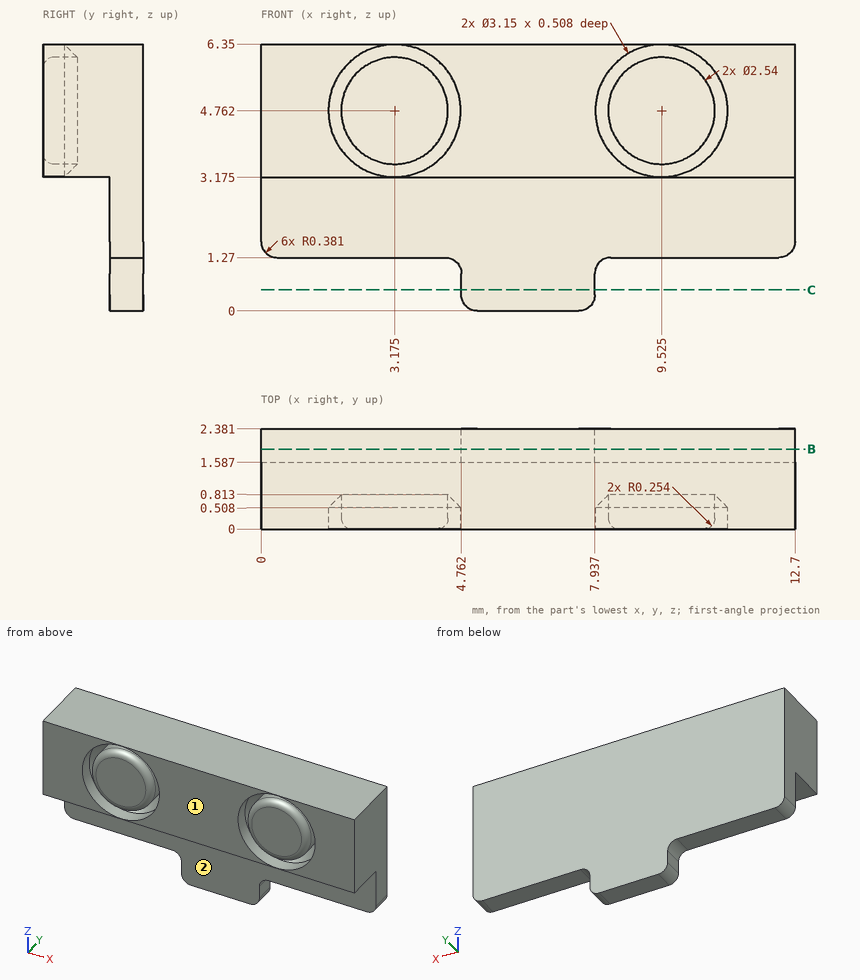
Could you check a few things on this drawing? It's one solid part, dimensions in mm from its lowest x, y, z. A direction names the side the tool comes from. Round coordinates to 2 decimals unless told otherwise and drop trailing zeros. Write each loop counter-clockwise with the first axis right and the second up, starting at its lowest first coordinate (ties: lowest second). Pieces come first, ordered by that corner, then holes. Notation, with made-up numbers: (-1.5, -22) -> (39.5, -22) arc R29 cw to (39.5, 12) -> close; hole circle Ø9 at (51, 56.5). An arc over 180 degrees is marked (long way). One line per question, with ' | ' between items. Start each with the question number.
1) On a 3-axis mill with a long thin cutter (end or side, diameter ignored), from which of +Z, -Z, +X, -X, +Y, -Y can I reach the whole of each face in a straight line? I mean the marked faces 1 and 2. Say none if no direction works.
2) Suppose I cut it at B-B on y = 1.9. Write out the boundary of the cut face in (x, z).
3) Suppose I cut it at C-C on z = 0.5. Write out the boundary of the cut face in (x, y).
4) I'm going to push flat-ended pins straight in: P1, Ø0.8, axis at x = 5, y = 0.5, coming from the -Z side (1 decimal); P2, Ø1, axis at x = 9, z = 1.5, coming from the -Y side; P3, Ø0.6, axis at y = 2, z = 0.5, coming from the +X side. Where does each tip first touch, or does it pass through?
5) I need wall thicknesses on line 1 (X direction, y = 1.65, z = 1) (1 decimal); line 2 (Y direction, x = 3, z = 2); line 3 (X direction, y = 2.1, z = 0.5). Which ranges of each line are inside material? Lowest first, please. Write a range as [from, to].
Return value:
1) face 1: +Z, -Z, +X, -X, -Y | face 2: -Z, +X, -X, -Y
2) outline: (0, 1.65) arc R0.38 ccw to (0.38, 1.27) -> (4.38, 1.27) arc R0.38 cw to (4.76, 0.89) -> (4.76, 0.38) arc R0.38 ccw to (5.14, 0) -> (7.56, 0) arc R0.38 ccw to (7.94, 0.38) -> (7.94, 0.89) arc R0.38 cw to (8.32, 1.27) -> (12.32, 1.27) arc R0.38 ccw to (12.7, 1.65) -> (12.7, 6.35) -> (0, 6.35) -> close
3) outline: (4.76, 1.59) -> (7.94, 1.59) -> (7.94, 2.38) -> (4.76, 2.38) -> close
4) P1: stops at z = 3.2 | P2: stops at y = 1.59 | P3: stops at x = 7.94
5) line 1: x = [4.7, 8] | line 2: y = [1.59, 2.38] | line 3: x = [4.76, 7.94]
